from build123d import *

# Parameters (mm, degrees)
F0_W     = 90
F0_H     = 6.258672
F0_R     = 2
F0_R_2   = 2.324227
F1_DEPTH = 5


with BuildPart() as f1:
    # F0 (on Top) → F1 (new body)
    with BuildSketch(Plane.XY):
        with Locations((1.716086, 0)):
            Rectangle(F0_W, F0_H)
        with Locations((-38.935287, 0)):
            Circle(F0_R, mode=Mode.SUBTRACT)
        Circle(F0_R_2, mode=Mode.SUBTRACT)
        with Locations((38.935287, 0)):
            Circle(F0_R, mode=Mode.SUBTRACT)
    extrude(amount=F1_DEPTH)


solid = f1.part
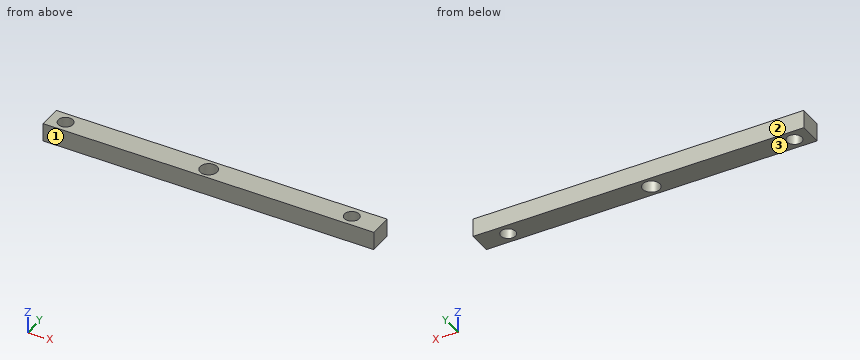
Geometry check sheet. Reference: the model listing, model coordinates, mm. Face numbers are marked on the shaded views. Coordinates: 2 decimals unless noted, no trailing zeros. Order: outer loops, then holes, each group sorted by start corner. A loop starts at its lowest first (then second) coordinate and runs counter-clockwise, first axis right, second up. Notation, with made-up numbers: (-30.75, -27.75) - (-5.75, -27.75) arc R29 cw to (-5.75, 1.25) - close; hole circle Ø7 at (28.5, 24.25). An arc over 180 degrees is marked (long way). One line per item, written item: value.
(1) Sectioned sample at A-A (x = 0). Enter the section's corners in (y, z).
Data:
outline: (-3.13, 0) - (-2.32, 0) - (-2.32, 5) - (-3.13, 5) - close; (2.32, 0) - (3.13, 0) - (3.13, 5) - (2.32, 5) - close
(2) Sectioned sample at B-B (y = 0). Enter the section's corners in (x, z).
Data:
outline: (-43.28, 0) - (-40.94, 0) - (-40.94, 5) - (-43.28, 5) - close; (-36.94, 0) - (-2.32, 0) - (-2.32, 5) - (-36.94, 5) - close; (2.32, 0) - (36.94, 0) - (36.94, 5) - (2.32, 5) - close; (40.94, 0) - (46.72, 0) - (46.72, 5) - (40.94, 5) - close
(3) Depth check by flat-ended pin: pin 1 Ø3.5 at (x, y) = (-38.94, 0) entering from -Z. Enter the tip coordinate at first touch or a pass-through.
Data:
pin 1: passes through
(4) Release check for a two-part mould opening along Y. For the marked faces 1, 2 and 3 record: +Y half, -Y half, draft (parallel to the pull), parting line (faces both ways), or undercut.
Data:
face 1: -Y half
face 2: +Y half
face 3: draft
(5) Thickness scan on probe 1 along X at (y, z) = (0.25, 4); probe 2 along Y at (x, z) = (0, 2); probe 3 along X at (y, z) = (-1, 4.7). Record the ranges inside material, lowest first. Write a range as from..to.
Data:
probe 1: x = -43.28..-40.92, -36.95..-2.31, 2.31..36.95, 40.92..46.72
probe 2: y = -3.13..-2.32, 2.32..3.13
probe 3: x = -43.28..-40.67, -37.2..-2.1, 2.1..37.2, 40.67..46.72
(6) Sectioned sample at C-C (z = 2.85). Enter the section's corners in (x, y).
Data:
outline: (-43.28, -3.13) - (46.72, -3.13) - (46.72, 3.13) - (-43.28, 3.13) - close; hole circle Ø4 at (-38.94, 0); hole circle Ø4.65 at (0, 0); hole circle Ø4 at (38.94, 0)
